```python
from build123d import *

# Parameters (mm, degrees)
SKETCH1_R           = 1
BOSS_EXTRUDE1_DEPTH = 7.5
CUT_EXTRUDE1_REACH  = 17.532
SKETCH2_W           = 4
SKETCH2_H           = 10
SKETCH2_W_2         = 10
SKETCH2_H_2         = 3


with BuildPart() as part:
    # Sketch1 → Boss-Extrude1 (new, symmetric)
    with BuildSketch(Plane.XY):
        with BuildLine():
            Line((-11, 4), (11, 4))
            ThreePointArc((11, 4), (13, 2), (11, 0))
            Line((11, 0), (-11, 0))
            ThreePointArc((-11, 0), (-13, 2), (-11, 4))
        make_face()
        with Locations((-11, 2)):
            Circle(SKETCH1_R, mode=Mode.SUBTRACT)
        with Locations((11, 2)):
            Circle(SKETCH1_R, mode=Mode.SUBTRACT)
    extrude(amount=BOSS_EXTRUDE1_DEPTH, both=True)

    # Sketch2 → Cut-Extrude1 (cut, up to next)
    with BuildSketch(Plane(origin=(0, 4, 0), x_dir=(1, 0, 0), z_dir=(0, 1, 0)), mode=Mode.PRIVATE) as cut_extrude1_sk1:
        with Locations((-11, 0)):
            Rectangle(SKETCH2_W, SKETCH2_H)
    cut_extrude1_tool1 = extrude(cut_extrude1_sk1.sketch, amount=-CUT_EXTRUDE1_REACH, mode=Mode.PRIVATE) & part.part
    # Sketch2 → Cut-Extrude1 (cut, up to next)
    with BuildSketch(Plane(origin=(0, 4, 0), x_dir=(1, 0, 0), z_dir=(0, 1, 0)), mode=Mode.PRIVATE) as cut_extrude1_sk2:
        with Locations((0, 6)):
            Rectangle(SKETCH2_W_2, SKETCH2_H_2)
    cut_extrude1_tool2 = extrude(cut_extrude1_sk2.sketch, amount=-CUT_EXTRUDE1_REACH, mode=Mode.PRIVATE) & part.part
    # Sketch2 → Cut-Extrude1 (cut, up to next)
    with BuildSketch(Plane(origin=(0, 4, 0), x_dir=(1, 0, 0), z_dir=(0, 1, 0)), mode=Mode.PRIVATE) as cut_extrude1_sk3:
        with Locations((0, -6)):
            Rectangle(SKETCH2_W_2, SKETCH2_H_2)
    cut_extrude1_tool3 = extrude(cut_extrude1_sk3.sketch, amount=-CUT_EXTRUDE1_REACH, mode=Mode.PRIVATE) & part.part
    # Sketch2 → Cut-Extrude1 (cut, up to next)
    with BuildSketch(Plane(origin=(0, 4, 0), x_dir=(1, 0, 0), z_dir=(0, 1, 0)), mode=Mode.PRIVATE) as cut_extrude1_sk4:
        with Locations((11, 0)):
            Rectangle(SKETCH2_W, SKETCH2_H)
    cut_extrude1_tool4 = extrude(cut_extrude1_sk4.sketch, amount=-CUT_EXTRUDE1_REACH, mode=Mode.PRIVATE) & part.part
    add(cut_extrude1_tool1.solids().sort_by_distance((-11, 4, 0))[0], mode=Mode.SUBTRACT)
    add(cut_extrude1_tool2.solids().sort_by_distance((0, 4, -6))[0], mode=Mode.SUBTRACT)
    add(cut_extrude1_tool3.solids().sort_by_distance((0, 4, 6))[0], mode=Mode.SUBTRACT)
    add(cut_extrude1_tool4.solids().sort_by_distance((11, 4, 0))[0], mode=Mode.SUBTRACT)


solid = part.part
```
Geometry: final body of the model. Coordinates: model frame, mm. A direction names the side the tool comes from. Round coordinates to 2 decimals unless told otherwise and drop trailing zeros. Order: outer loops, then holes, each group sorted by start corner. A loop starts at its lowest first (then second) coordinate and runs counter-clockwise, first axis right, second up. Notation, with made-up numbers: (57.25, -36) -> (91.25, -36) arc R27 cw to (91.25, -14) -> close; hole circle Ø2 at (-5, -7). An arc over 180 degrees is marked (long way). Use one line per item in the form item = value.
(1) Section D-D on z = -3.5. Return loops of the section in (x, y), and give its area (3 significant figures).
Results list:
outline = (-9, 0) -> (9, 0) -> (9, 4) -> (-9, 4) -> close
area = 72.0 mm^2
(2) First-contact query: pin 1 Ø2 at (y, z) = (1.5, 0) entering from -X; pin 2 Ø1.5 at (y, z) = (3, -5.5) entering from +X; pin 3 Ø2 at (x, y) = (-2.5, 1.5) entering from +Z. Flat tips, straight axial feed; report the tip coordinate or a pass-through.
Results list:
pin_1 = -9
pin_2 = 12.98
pin_3 = 4.5
(3) Ray query, probe 1 along X at (y, z) = (2, 6.95); probe 2 along Y at (x, z) = (-11, 6.3); probe 3 along Z at (x, y) = (-12, 0.8). Return the intervals inside material, ascending. Write a range as [from, to].
Results list:
probe_1 = [-13, -12], [-10, -5], [5, 10], [12, 13]
probe_2 = [0, 1], [3, 4]
probe_3 = [-7.5, -5], [5, 7.5]
(4) Draft query along Y for faces 4 (the face through (-11.8, 1.4, 6.2)), 5 (the face through (13, 2, -6)), 6 (the face through (8, 2, -7.5)). Return one class per face: pulls with the +Y half, pulls with the -Y half, needs draft (parallel to the pull), parting line crosses it, or undercut.
Results list:
face_4 = undercut
face_5 = parting line crosses it
face_6 = needs draft
(5) Section C-C on y = 1.7. Count the separate pieces of the cut face and the enclosed holes in it, and give its area (3 significant figures).
Results list:
separate_pieces = 5
enclosed_holes = 0
area = 231 mm^2
(6) Access query for faces 1 (the face through (5, 2, -6)), 2 (the face through (-9, 2, 0)), 3 (the face through (10, 1, -5)). Directions: +Z, -Z, +X, -X, +Y, -Y. A direction counts if a zero-diameter tool reaches every point of the face in a straight line with its end or side. Return the directions, or none.
Results list:
face_1 = -Z, +Y, -Y
face_2 = -X, +Y, -Y
face_3 = +X, +Y, -Y
(7) Section A-A on z = -5.75. Return loops of the section in (x, y), and give its area (3 significant figures).
Results list:
outline = (-11, 0) -> (-5, 0) -> (-5, 4) -> (-11, 4) arc R2 ccw to start; (5, 0) -> (11, 0) arc R2 ccw to (11, 4) -> (5, 4) -> close; hole circle Ø2 at (-11, 2); hole circle Ø2 at (11, 2)
area = 54.3 mm^2
(8) Section B-B on x = 11.5. Return loops of the section in (y, z).
Results list:
outline = (0.06, -7.5) -> (1.13, -7.5) -> (1.13, -5) -> (0.06, -5) -> close; (0.06, 5) -> (1.13, 5) -> (1.13, 7.5) -> (0.06, 7.5) -> close; (2.87, -7.5) -> (3.94, -7.5) -> (3.94, -5) -> (2.87, -5) -> close; (2.87, 5) -> (3.94, 5) -> (3.94, 7.5) -> (2.87, 7.5) -> close
